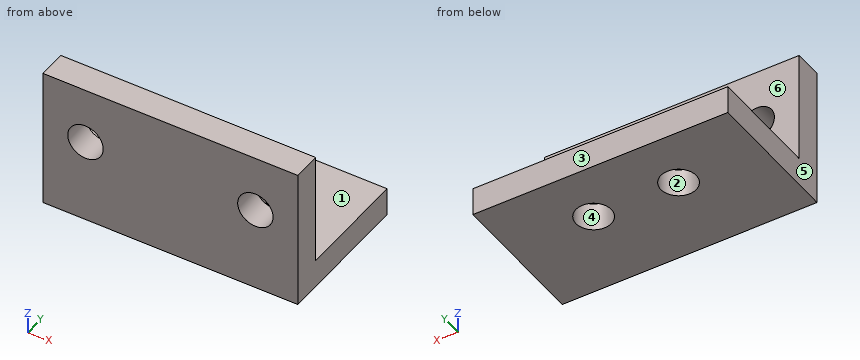
```python
from build123d import *

# Parameters (mm, degrees)
SKETCH1_W           = 25.4
SKETCH1_H           = 6.35
SKETCH1_W_2         = 6.35
SKETCH1_H_2         = 31.75
BOSS_EXTRUDE1_DEPTH = 57.15
CUT_EXTRUDE1_REACH  = 8.35
SKETCH2_R           = 3.96875
CUT_EXTRUDE2_REACH  = 8.35
SKETCH3_R           = 3.96875


with BuildPart() as part:
    # Sketch1 → Boss-Extrude1 (new body)
    with BuildSketch(Plane(origin=(0, 0, 0), x_dir=(0, 0, -1), z_dir=(1, 0, 0))):
        with Locations((-19.05, 3.175)):
            Rectangle(SKETCH1_W, SKETCH1_H)
        with Locations((-3.175, 15.875)):
            Rectangle(SKETCH1_W_2, SKETCH1_H_2)
    extrude(amount=BOSS_EXTRUDE1_DEPTH)

    # Sketch2 → Cut-Extrude1 (cut, up to next)
    with BuildSketch(Plane.XY.offset(6.35), mode=Mode.PRIVATE) as cut_extrude1_sk1:
        with Locations((19.05, 19.05)):
            Circle(SKETCH2_R)
    cut_extrude1_tool1 = extrude(cut_extrude1_sk1.sketch, amount=-CUT_EXTRUDE1_REACH, mode=Mode.PRIVATE) & part.part
    add(cut_extrude1_tool1.solids().sort_by_distance((19.05, 19.05, 6.35))[0], mode=Mode.SUBTRACT)
    # Sketch2 → Cut-Extrude1 (cut, up to next)
    with BuildSketch(Plane.XY.offset(6.35), mode=Mode.PRIVATE) as cut_extrude1_sk2:
        with Locations((38.1, 19.05)):
            Circle(SKETCH2_R)
    cut_extrude1_tool2 = extrude(cut_extrude1_sk2.sketch, amount=-CUT_EXTRUDE1_REACH, mode=Mode.PRIVATE) & part.part
    add(cut_extrude1_tool2.solids().sort_by_distance((38.1, 19.05, 6.35))[0], mode=Mode.SUBTRACT)

    # Sketch3 → Cut-Extrude2 (cut, up to next)
    with BuildSketch(Plane(origin=(0, 6.35, 0), x_dir=(1, 0, 0), z_dir=(0, 1, 0)), mode=Mode.PRIVATE) as cut_extrude2_sk1:
        with Locations((9.525, -19.05)):
            Circle(SKETCH3_R)
    cut_extrude2_tool1 = extrude(cut_extrude2_sk1.sketch, amount=-CUT_EXTRUDE2_REACH, mode=Mode.PRIVATE) & part.part
    add(cut_extrude2_tool1.solids().sort_by_distance((9.525, 6.35, 19.05))[0], mode=Mode.SUBTRACT)
    # Sketch3 → Cut-Extrude2 (cut, up to next)
    with BuildSketch(Plane(origin=(0, 6.35, 0), x_dir=(1, 0, 0), z_dir=(0, 1, 0)), mode=Mode.PRIVATE) as cut_extrude2_sk2:
        with Locations((47.625, -19.05)):
            Circle(SKETCH3_R)
    cut_extrude2_tool2 = extrude(cut_extrude2_sk2.sketch, amount=-CUT_EXTRUDE2_REACH, mode=Mode.PRIVATE) & part.part
    add(cut_extrude2_tool2.solids().sort_by_distance((47.625, 6.35, 19.05))[0], mode=Mode.SUBTRACT)


solid = part.part
```
Input: part model. Units: mm. Frame: model coordinates. Face numbers are marked on the shaded views. A direction names the side the tool comes from. Give positions to 0.01 mm unless a question says otherwise; leave off trailing zeros. Order: outer loops, then holes, each group sorted by start corner. A loop starts at its lowest first (then second) coordinate and runs counter-clockwise, first axis right, second up. Notation, with made-up numbers: M 70.25,26.5 L 120.25,26.5 A21 cw 120.25,47.5 Z; hole C 67,85.5 d6. An arc over 180 degrees is marked long. One line per question, with ' | ' between items. Start each with the question number.
1. Section query C-C (y = 19.05). Return the cut outline in (x, z), and give its area (3 significant figures).
2. Pull-direction query (Y, two-part tool) for the marked faces 1, 2, 3 and 4; classes: released by +Y, released by -Y, zero draft, split by the parting line, or undercut.
3. Section query A-A (z = 19.05). Return the cut outline in (x, y).
4. First-contact query: pin 1 Ø7.5 at (x, z) = (27, 23) entering from +Y; pin 2 Ø7 at (x, y) = (38.1, 19.05) entering from -Z; pin 3 Ø7.5 at (x, y) = (39, 14) entering from +Z. Flat tips, straight axial feed; report the tip coordinate or a pass-through.
5. Access query for the marked faces 5 and 6. Directions: +Z, -Z, +X, -X, +Y, -Y. A direction counts if a zero-diameter tool reaches every point of the face in a straight line with its end or side. Return the directions, or none.
6. Section query B-B (x = 19.05). Return the cut outline in (y, z), and give its area (4 significant figures).
7. Section query D-D (x = 32.5). Return the cut outline in (y, z), and give its area (3 significant figures).
8. Material intervals for probe 1 along X at (y, z) = (4, 19); probe 2 along X at (y, z) = (19, 3); probe 3 along Y at (x, z) = (19, 1), sorted ascending. Write a range as [from, to].
Here are the results:
1) outline: M 0,0 L 15.08,0 L 15.08,6.35 L 0,6.35 Z; M 23.02,0 L 34.13,0 L 34.13,6.35 L 23.02,6.35 Z; M 42.07,0 L 57.15,0 L 57.15,6.35 L 42.07,6.35 Z | area: 262 mm²
2) face 1: zero draft | face 2: undercut | face 3: released by +Y | face 4: undercut
3) outline: M 0,0 L 5.56,0 L 5.56,6.35 L 0,6.35 Z; M 13.49,0 L 43.66,0 L 43.66,6.35 L 13.49,6.35 Z; M 51.59,0 L 57.15,0 L 57.15,6.35 L 51.59,6.35 Z
4) pin 1: y = 6.35 | pin 2: through | pin 3: z = 6.35
5) face 5: +Z, -Z, -X, +Y, -Y | face 6: +Z, +X, -X, +Y
6) outline: M 0,0 L 15.08,0 L 15.08,6.35 L 6.35,6.35 L 6.35,31.75 L 0,31.75 Z; M 23.02,0 L 31.75,0 L 31.75,6.35 L 23.02,6.35 Z | area: 312.5 mm²
7) outline: M 0,0 L 31.75,0 L 31.75,6.35 L 6.35,6.35 L 6.35,31.75 L 0,31.75 Z | area: 363 mm²
8) probe 1: [0, 5.56], [13.49, 43.66], [51.59, 57.15] | probe 2: [0, 15.08], [23.02, 34.13], [42.07, 57.15] | probe 3: [0, 15.08], [23.02, 31.75]
